```python
from build123d import *

# Parameters (mm, degrees)
CUT_EXTRUDE1_START         = -11
CUT_EXTRUDE1_OUTLINE_R     = 25
CUT_EXTRUDE1_OUTLINE_R_2   = 10.5
CUT_EXTRUDE1_DEPTH         = 11
CUT_EXTRUDE1_2_OUTLINE_R   = 10.5
CUT_EXTRUDE1_2_OUTLINE_R_2 = 1.6
CUT_EXTRUDE1_2_OUTLINE_R_3 = 3.16810248
CUT_EXTRUDE1_2_DEPTH       = 8
SKETCH2_R                  = 30
BOSS_EXTRUDE1_DEPTH        = 2.5
BOSS_EXTRUDE2_START        = -2.5
SKETCH3_R                  = 30
BOSS_EXTRUDE2_DEPTH        = 2.5
SKETCH4_R                  = 11.25
CUT_EXTRUDE2_DEPTH         = 3
CUT_EXTRUDE3_START         = -3
SKETCH5_R                  = 3.16810248
CUT_EXTRUDE3_DEPTH         = 3
CUT_EXTRUDE4_START         = -3
SKETCH7_R                  = 11.25
CUT_EXTRUDE4_DEPTH         = 3


with BuildPart() as part:
    # Cut-Extrude1: read off the stored shape, not the designer's step
    # Cut-Extrude1 outline → Cut-Extrude1 (new body)
    with BuildSketch(Plane.XY.offset(11).offset(CUT_EXTRUDE1_START)):
        Circle(CUT_EXTRUDE1_OUTLINE_R)
        Circle(CUT_EXTRUDE1_OUTLINE_R_2, mode=Mode.SUBTRACT)
    extrude(amount=CUT_EXTRUDE1_DEPTH)

    # Cut-Extrude1 2 outline → Cut-Extrude1 2 (add)
    with BuildSketch(Plane.XY.offset(11).offset(CUT_EXTRUDE1_START)):
        Circle(CUT_EXTRUDE1_2_OUTLINE_R)
        with Locations((0, -7)):
            Circle(CUT_EXTRUDE1_2_OUTLINE_R_2, mode=Mode.SUBTRACT)
        with Locations((-7, 0)):
            Circle(CUT_EXTRUDE1_2_OUTLINE_R_2, mode=Mode.SUBTRACT)
        Circle(CUT_EXTRUDE1_2_OUTLINE_R_3, mode=Mode.SUBTRACT)
        with Locations((7, 0)):
            Circle(CUT_EXTRUDE1_2_OUTLINE_R_2, mode=Mode.SUBTRACT)
        with Locations((0, 7)):
            Circle(CUT_EXTRUDE1_2_OUTLINE_R_2, mode=Mode.SUBTRACT)
    extrude(amount=CUT_EXTRUDE1_2_DEPTH)

    # Sketch2 → Boss-Extrude1 (add)
    with BuildSketch(Plane.XY.offset(11)):
        Circle(SKETCH2_R)
    extrude(amount=-BOSS_EXTRUDE1_DEPTH)

    # Sketch3 → Boss-Extrude2 (add)
    with BuildSketch(Plane(origin=(0, 0, 0), x_dir=(-1, 0, 0), z_dir=(0, 0, -1)).offset(BOSS_EXTRUDE2_START)):
        with Locations(Location((0, 0, 0), (0, 0, 180))):
            Circle(SKETCH3_R)
    extrude(amount=BOSS_EXTRUDE2_DEPTH)

    # Sketch4 → Cut-Extrude2 (cut)
    with BuildSketch(Plane.XY.offset(11)):
        Circle(SKETCH4_R)
    extrude(amount=-CUT_EXTRUDE2_DEPTH, mode=Mode.SUBTRACT)

    # Sketch5 → Cut-Extrude3 (cut)
    with BuildSketch(Plane.XY.offset(2.5).offset(CUT_EXTRUDE3_START)):
        Circle(SKETCH5_R)
    extrude(amount=CUT_EXTRUDE3_DEPTH, mode=Mode.SUBTRACT)

    # Sketch7 → Cut-Extrude4 (cut)
    with BuildSketch(Plane(origin=(0, 0, 0), x_dir=(-1, 0, 0), z_dir=(0, 0, -1)).offset(CUT_EXTRUDE4_START)):
        with Locations(Location((0, 0, 0), (0, 0, 180))):
            Circle(SKETCH7_R)
    extrude(amount=CUT_EXTRUDE4_DEPTH, mode=Mode.SUBTRACT)


solid = part.part
```
Can you work these out from the model? Positions are in its coordinate system, mm. A direction names the side the tool comes from. Coordinates: 2 decimals unless noted, no trailing zeros. Loops run counter-clockwise (first coordinate to the right, second up) from the corner with the lowest first, then second, coordinate; pieces in that order, holes last. Notation, with made-up numbers: M -36.75,-28.75 L -31.75,-28.75 A14 cw -31.75,-9.75 Z; hole C -29,77.25 d11. An arc over 180 degrees is marked long. Put each result on its own line as item: value. Start each with the question number.
(1) We'd pull the mould along X, two halves only. Please class faces 4 (the face through (2, -3, 3)), 5 (the face through (23.846, 7.509, 5.458)), 6 (the face through (-7, 25, 8.5)): +X half, -X half, draft (parallel to the pull), parting line (faces both ways), or undercut.
(2) I need wall thicknesses on probe 1 along X at (y, z) = (0, 4.85); probe 2 along Z at (x, y) = (-26, -10). Which ranges of each line are inside material? Lowest first, please.
(3) Imagine slicing it at A-A on y = 7. List the corners of the cut face in (x, z) for me.
(4) Will these pins go through, and if not, where does the flat tip stop? pin 1 Ø2 at (x, z) = (19, 9.5) entering from -Y; pin 2 Ø1.5 at (x, z) = (-2, 1.5) entering from +Y; pin 3 Ø2 at (x, y) = (7.5, 5) entering from +Z; pin 4 Ø1.9 at (x, y) = (0, -7) entering from +Z.
(5) Imagine slicing it at C-C on z = 10. List the corners of the cut face in (x, y) for me, and give its area (3 significant figures).
(6) Imagine slicing it at D-D on x = 17.5. List the corners of the cut face in (y, z) for me, and give its area (3 significant figures).
(7) Which directions (+Z, -Z, +X, -X, +Y, -Y) give clear straight access to the entire face, cutting with the end or side of a thin tool? Please do faces 1 (the face through (-7, -25, 2.5)), 2 (the face through (5.19, -9.98, 9.52)), 3 (the face through (5.19, 9.98, 1.52)).
Worked answers:
1. face 4: undercut
1. face 5: parting line
1. face 6: draft
2. probe 1: x = -25 to -8.6, -5.4 to -3.17, 3.17 to 5.4, 8.6 to 25
2. probe 2: z = 0 to 2.5, 8.5 to 11
3. outline: M -29.17,0 L -8.81,0 L -8.81,3 L -1.6,3 L -1.6,8 L -8.81,8 L -8.81,11 L -29.17,11 L -29.17,8.5 L -24,8.5 L -24,2.5 L -29.17,2.5 Z; M 1.6,3 L 8.81,3 L 8.81,0 L 29.17,0 L 29.17,2.5 L 24,2.5 L 24,8.5 L 29.17,8.5 L 29.17,11 L 8.81,11 L 8.81,8 L 1.6,8 Z
4. pin 1: stops at y = -24
4. pin 2: stops at y = 29.97
4. pin 3: stops at z = 8
4. pin 4: passes through
5. outline: C 0,0 d60; hole C 0,0 d22.5
5. area: 2,430 mm2
6. outline: M -24.37,0 L 24.37,0 L 24.37,2.5 L 17.85,2.5 L 17.85,8.5 L 24.37,8.5 L 24.37,11 L -24.37,11 L -24.37,8.5 L -17.85,8.5 L -17.85,2.5 L -24.37,2.5 Z
6. area: 458 mm2
7. face 1: none
7. face 2: +Z
7. face 3: -Z
